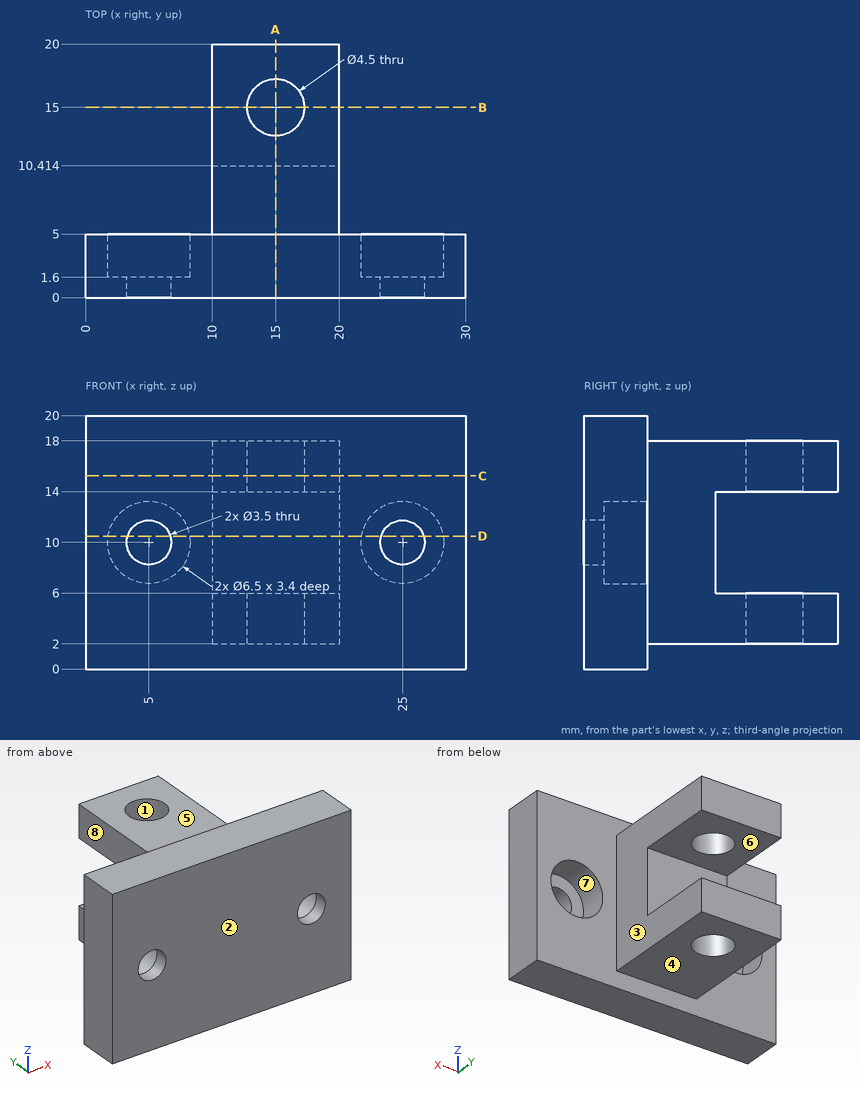
The figure shows three views and two pictorial views of one solid part (mm, origin at its lowest corner). Answer the questions. A direction names the side the tool comes from. Coordinates: 2 decimals unless noted, no trailing zeros. Loops run counter-clockwise (first coordinate to the right, second up) from the corner with the lowest first, then second, coordinate; pieces in that order, holes last. Notation, with made-up numbers: (64.5, -22.5) - (94.5, -22.5) arc R19 ccw to (94.5, -16.5) - close; hole circle Ø2 at (45.25, -10). An arc over 180 degrees is marked (long way). Write item = value, one per line.
1) Find the intervals of material crossed by line 1 along X through (y, z) = (2.75, 10); line 2 along X through (y, z) = (1.25, 10); line 3 along Y through (x, z) = (15, 16.95), in increasing order.
Responses:
line_1 = 0 to 1.75, 8.25 to 21.75, 28.25 to 30
line_2 = 0 to 3.25, 6.75 to 23.25, 26.75 to 30
line_3 = 0 to 12.75, 17.25 to 20
2) Section A-A (x = 15) is taken. Determine the outline of the cut face in (y, z).
Responses:
outline = (0, 0) - (5, 0) - (5, 2) - (12.75, 2) - (12.75, 6) - (10.41, 6) - (10.41, 14) - (12.75, 14) - (12.75, 18) - (5, 18) - (5, 20) - (0, 20) - close; (17.25, 2) - (20, 2) - (20, 6) - (17.25, 6) - close; (17.25, 14) - (20, 14) - (20, 18) - (17.25, 18) - close
3) Each of these flat-tipped pins is pushed along its axis until it touches: P1, Ø10, axis at x = 10, y = 14, coming from the -Z side; P2, Ø4, axis at x = 14, z = 9.5, coming from the +Y side; P3, Ø7, axis at x = 6, z = 11.5, coming from the +Y side; P4, Ø3, axis at x = 25, z = 10, coming from the +Y side. Where does it stop, or does it pass through?
Responses:
P1 = 2
P2 = 10.41
P3 = 5
P4 = through
4) Section C-C (z = 15.25) is taken. Determine the outline of the cut face in (x, y), plus the area to 3 significant figures.
Responses:
outline = (0, 0) - (30, 0) - (30, 5) - (20, 5) - (20, 20) - (10, 20) - (10, 5) - (0, 5) - close; hole circle Ø4.5 at (15, 15)
area = 284 mm^2
5) Which of the six approach directions +Z, -Z, +X, -X, +Y, -Y give full straight-line access (tool end or side, diameter ignored) to the marked faces 4, 5, 6, 7 and 8?
Responses:
face_4 = -Z, +X, -X, +Y
face_5 = +Z, +X, -X, +Y
face_6 = +X, -X, +Y
face_7 = +Y
face_8 = +Z, -Z, -X, +Y
6) Section D-D (z = 10.5) is taken. Determine the outline of the cut face in (x, y).
Responses:
outline = (0, 0) - (3.32, 0) - (3.32, 1.6) - (1.79, 1.6) - (1.79, 5) - (0, 5) - close; (6.68, 0) - (23.32, 0) - (23.32, 1.6) - (21.79, 1.6) - (21.79, 5) - (20, 5) - (20, 10.41) - (10, 10.41) - (10, 5) - (8.21, 5) - (8.21, 1.6) - (6.68, 1.6) - close; (26.68, 0) - (30, 0) - (30, 5) - (28.21, 5) - (28.21, 1.6) - (26.68, 1.6) - close
7) Determine the mould class of the marked faces 1, 2 and 3 for opening direction Y: pulls with the +Y half, pulls with the -Y half, needs draft (parallel to the pull), parting line crosses it, or undercut.
Responses:
face_1 = undercut
face_2 = pulls with the -Y half
face_3 = needs draft
8) Section B-B (y = 15) is taken. Determine the outline of the cut face in (x, z).
Responses:
outline = (10, 2) - (12.75, 2) - (12.75, 6) - (10, 6) - close; (10, 14) - (12.75, 14) - (12.75, 18) - (10, 18) - close; (17.25, 2) - (20, 2) - (20, 6) - (17.25, 6) - close; (17.25, 14) - (20, 14) - (20, 18) - (17.25, 18) - close
